CAD build for the part. Positions are in the model's coordinates, mm. A direction names the side the tool comes from. Give positions to 0.01 mm unless a question says otherwise; leave off trailing zeros. Loops run counter-clockwise (first coordinate to the right, second up) from the corner with the lowest first, then second, coordinate; pieces in that order, holes last. Notation, with made-up numbers: (75.5, -36) -> (108.5, -36) arc R14 ccw to (108.5, -30) -> close; hole circle Ø5 at (40, -5). An arc over 180 degrees is marked (long way). Write each question's results on one line, items separated by ' | '. Start each with the question number.
```python
from build123d import *

# Parameters (mm, degrees)
IZIM1_W                     = 10.606601718
IZIM1_H                     = 10.606601718
Y_KSEKLIK_EKSTR_ZYON1_DEPTH = 2
IZIM2_R                     = 3.95
Y_KSEKLIK_EKSTR_ZYON2_DEPTH = 25
KES_EKSTR_ZYON1_DEPTH       = 10
IZIM5_R                     = 1.6
KES_EKSTR_ZYON3_DEPTH       = 26
IZIM8_W                     = 5
IZIM8_H                     = 13.621024602
KES_EKSTR_ZYON4_DEPTH       = 29.022312538
SKETCH2_R                   = 3
BOSS_EXTRUDE1_DEPTH         = 17


with BuildPart() as part:
    # Çizim1 → Yükseklik-Ekstrüzyon1 (new body)
    with BuildSketch(Plane.XY):
        Rectangle(IZIM1_W, IZIM1_H)
    extrude(amount=Y_KSEKLIK_EKSTR_ZYON1_DEPTH)

    # Çizim2 → Yükseklik-Ekstrüzyon2 (add)
    with BuildSketch(Plane(origin=(0, 0, 0), x_dir=(-1, 0, 0), z_dir=(0, 0, -1))):
        with Locations(Location((0, 0, 0), (0, 0, 180))):
            Circle(IZIM2_R)
    extrude(amount=Y_KSEKLIK_EKSTR_ZYON2_DEPTH)

    # Çizim3 → Kes-Ekstrüzyon1 (cut)
    with BuildSketch(Plane.XY.offset(2)):
        with BuildLine():
            Line((-2, -1.959591794), (-2, 1.959591794))
            ThreePointArc((-2, 1.959591794), (0, 2.8), (2, 1.959591794))
            Line((2, 1.959591794), (2, -1.959591794))
            ThreePointArc((2, -1.959591794), (0, -2.8), (-2, -1.959591794))
        make_face()
    extrude(amount=-KES_EKSTR_ZYON1_DEPTH, mode=Mode.SUBTRACT)

    # Çizim5 → Kes-Ekstrüzyon3 (cut, symmetric)
    with BuildSketch(Plane(origin=(0, 0, 0), x_dir=(0, 0, -1), z_dir=(1, 0, 0))):
        with Locations((4.6, 0)):
            Circle(IZIM5_R)
        with Locations((17.6, 0)):
            Circle(IZIM5_R)
    extrude(amount=KES_EKSTR_ZYON3_DEPTH, both=True, mode=Mode.SUBTRACT)

    # Çizim8 → Kes-Ekstrüzyon4 (cut, through all)
    with BuildSketch(Plane(origin=(0, 0, -25), x_dir=(-1, 0, 0), z_dir=(0, 0, -1))):
        with Locations((-5.8, 0)):
            Rectangle(IZIM8_W, IZIM8_H)
    extrude(amount=-KES_EKSTR_ZYON4_DEPTH, mode=Mode.SUBTRACT)

    # Sketch2 → Boss-Extrude1 (add)
    with BuildSketch(Plane(origin=(0, 0, -25), x_dir=(-1, 0, 0), z_dir=(0, 0, -1))):
        Circle(SKETCH2_R)
    extrude(amount=BOSS_EXTRUDE1_DEPTH)


solid = part.part
```
Q1. Saw through at D-D, the plane x = 2.5. List the corners of the cut face in (y, z), then the cut area to 3 significant figures.
Q2. Drop flat-ended pins along their axis: pin 1 (1.5 mm diameter, centred on y = 2.5, z = -3, fed in from -X); pin 2 (5 mm diameter, centred on y = 2, z = -37, fed in from +X); pin 3 (5 mm diameter, centred on y = 0, z = -4.6, fed in from -X); pin 4 (3 mm diameter, centred on y = 0, z = -17.6, fed in from -X). Give the stop position or say it passes through.
Q3. Wall check: L1, parallel to Z at x = 2.4, y = 0; L2, parallel to Z at x = -1, y = 0; L3, parallel to Y at x = 0, z = -14.5. Give the ranges that are in metal, low to high.
Q4. Saw through at B-B, the plane z = -4.6. List the corners of the cut face in (x, y).
Q5. Saw through at A-A, the plane y = 0. List the corners of the cut face in (x, z).
Q6. Which spindle directions (+Z, -Z, +X, -X, +Y, -Y) get a long thin tool onto all of the face, cutting with end or side? Do faces 1 (the face through (-1, -5.303, 1)), 2 (the face through (0, -2.8, -2.9)), 3 (the face through (-3, -1, -25)). Say none if no direction does.
Q7. Mould opens along Z. For faces 4 (the face through (3, 0, -3)), 5 (the face through (0, 0, -8)), 6 (the face through (-5.303, 0, 1)) say: pulls with the +Z half, pulls with the -Z half, needs draft (parallel to the pull), parting line crosses it, or undercut.
Q8. Saw through at C-C, the plane x = -1.25. List the corners of the cut face in (y, z), then the cut area to 3 significant figures.
Answer block:
1) outline: (-5.3, 0) -> (-3.06, 0) -> (-3.06, -25) -> (-1.66, -25) -> (-1.66, -42) -> (1.66, -42) -> (1.66, -25) -> (3.06, -25) -> (3.06, 0) -> (5.3, 0) -> (5.3, 2) -> (-5.3, 2) -> close; hole circle Ø3.2 at (0, -17.6); hole circle Ø3.2 at (0, -4.6) | area: 214 mm2
2) pin 1: stops at x = -3.54 | pin 2: stops at x = 3 | pin 3: stops at x = -3.95 | pin 4: passes through
3) L1: z = -42 to -19.2, -16 to -6.2, -3 to 2 | L2: z = -42 to -19.2, -16 to -8 | L3: y = -3.95 to 3.95
4) outline: (-3.61, -1.6) arc R3.95 ccw to (3.3, -2.17) -> (3.3, -1.6) -> (2, -1.6) -> (2, -1.96) arc R2.8 cw to (-2, -1.96) -> (-2, -1.6) -> close; (-3.61, 1.6) -> (-2, 1.6) -> (-2, 1.96) arc R2.8 cw to (2, 1.96) -> (2, 1.6) -> (3.3, 1.6) -> (3.3, 2.17) arc R3.95 ccw to start
5) outline: (-5.3, 0) -> (-3.95, 0) -> (-3.95, -3) -> (-2, -3) -> (-2, 2) -> (-5.3, 2) -> close; (-3.95, -25) -> (-3, -25) -> (-3, -42) -> (3, -42) -> (3, -25) -> (3.3, -25) -> (3.3, -19.2) -> (-3.95, -19.2) -> close; (-3.95, -16) -> (3.3, -16) -> (3.3, -6.2) -> (2, -6.2) -> (2, -8) -> (-2, -8) -> (-2, -6.2) -> (-3.95, -6.2) -> close; (2, -3) -> (3.3, -3) -> (3.3, 2) -> (2, 2) -> close
6) face 1: +Z, -Z, +X, -X, -Y | face 2: +Z | face 3: -Z
7) face 4: undercut | face 5: pulls with the +Z half | face 6: needs draft
8) outline: (-5.3, 0) -> (-3.75, 0) -> (-3.75, -25) -> (-2.73, -25) -> (-2.73, -42) -> (2.73, -42) -> (2.73, -25) -> (3.75, -25) -> (3.75, 0) -> (5.3, 0) -> (5.3, 2) -> (2.51, 2) -> (2.51, -8) -> (-2.51, -8) -> (-2.51, 2) -> (-5.3, 2) -> close; hole circle Ø3.2 at (0, -17.6) | area: 243 mm2
